Study the drawing (mm; zero at the part's minimum x, y, z) and answer. A direction names the side the tool comes from. Coordinates: 2 decimals unless noted, no trailing zeros. Loops run counter-clockwise (first coordinate to the right, second up) from the corner with the lowest first, then second, coordinate; pieces in that order, holes last. Notation, with made-up numbers: (4, 49.25) - (21, 49.25) arc R21 cw to (21, 56.25) - close; hole circle Ø8 at (71, 41). An arc over 180 degrees is marked (long way). Put each result on its own line as item: value.
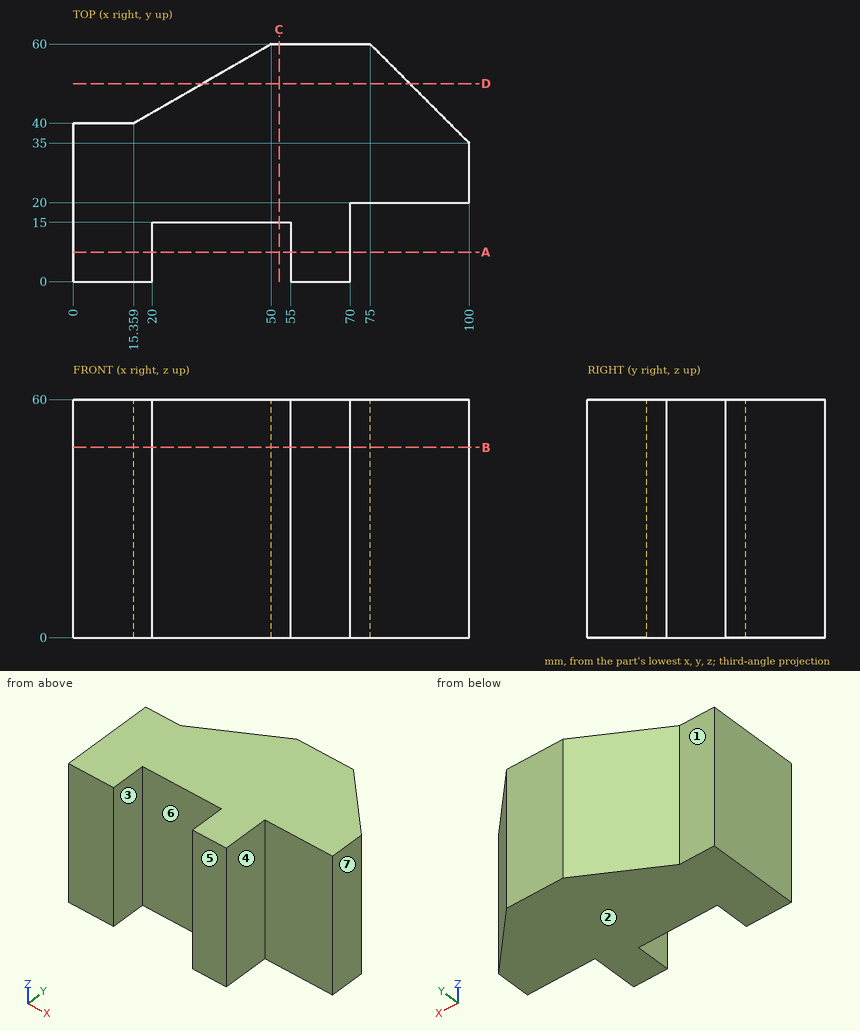
1) The part is cut by section D-D (y = 50). Give the vertices of the cut face in (x, z), and give its area (3 significant figures).
Found:
outline: (32.68, 0) - (85, 0) - (85, 60) - (32.68, 60) - close
area: 3,140 mm^2
2) The part is cut by section B-B (z = 48). Give the vertices of the cut face in (x, y).
Found:
outline: (0, 0) - (20, 0) - (20, 15) - (55, 15) - (55, 0) - (70, 0) - (70, 20) - (100, 20) - (100, 35) - (75, 60) - (50, 60) - (15.36, 40) - (0, 40) - close
3) The part is cut by section A-A (y = 7.5). Give the vertices of the cut face in (x, z).
Found:
outline: (0, 0) - (20, 0) - (20, 60) - (0, 60) - close; (55, 0) - (70, 0) - (70, 60) - (55, 60) - close
4) For a pull along X with two mould halves and no side action, classify the marked faces 5, 6 and 7 as pulls with the +X half, pulls with the -X half, needs draft (parallel to the pull), parting line crosses it, or undercut.
Found:
face 5: needs draft
face 6: undercut
face 7: pulls with the +X half
5) The part is cut by section C-C (x = 52). Give the vertices of the cut face in (y, z), and give its area (3 significant figures).
Found:
outline: (15, 0) - (60, 0) - (60, 60) - (15, 60) - close
area: 2,700 mm^2
6) Straight lines are drawn through the part: L1, parallel to X at y = 13, z = 45.5; L2, parallel to X at y = 18.5, z = 32; L3, parallel to Y at x = 87, z = 12. For each, find the intervals that lie inside material, in ascending order. Write a range as [from, to].
Found:
L1: x = [0, 20], [55, 70]
L2: x = [0, 70]
L3: y = [20, 48]
7) Each of these flat-tipped pins is pushed along its axis until it touches: pin 1 (7.5 mm diameter, centred on x = 11, z = 27, fed in from +Y); pin 2 (8 mm diameter, centred on x = 80.5, z = 27, fed in from +Y); pin 3 (9 mm diameter, centred on x = 85.5, z = 37.5, fed in from -Y). Where does it stop, or does it pass through?
Found:
pin 1: stops at y = 40
pin 2: stops at y = 58.5
pin 3: stops at y = 20
8) For the marked faces 1, 2, 3 and 4, determine the directions among +Z, -Z, +X, -X, +Y, -Y from which every point of the face is accessible in a straight line to the end or side of a thin tool.
Found:
face 1: +Z, -Z, -X, +Y
face 2: -Z, +X, -X, +Y, -Y
face 3: +Z, -Z, -Y
face 4: +Z, -Z, +X, -Y
